```python
from build123d import *

# Parameters (mm, degrees)
F2_W     = 50.8
F2_H     = 76.2
F2_W_2   = 45.72
F2_H_2   = 71.12
F3_DEPTH = 50.8
F4_W     = 50.8
F4_H     = 76.2
F5_DEPTH = 2.54
F8_D     = 12.7
F8_DEPTH = 5.08
F8_TIP   = 3.8154649308


# Not quite as in the source:
# - a variable given as a bare number and used for a length is read in inches; the dataset says mm whatever the document's units were


with BuildPart() as f3:
    # F2 (on Top) → F3 (new body)
    with BuildSketch(Plane.XY):
        with Locations((25.4, 38.1)):
            Rectangle(F2_W, F2_H)
        with Locations((25.4, 38.1)):
            Rectangle(F2_W_2, F2_H_2, mode=Mode.SUBTRACT)
    extrude(amount=F3_DEPTH)

    # F4 (on Top) → F5 (join)
    with BuildSketch(Plane.XY):
        with Locations((25.4, 38.1)):
            Rectangle(F4_W, F4_H)
    extrude(amount=F5_DEPTH)

    # F8
    with Locations(Plane(origin=(0, 0, 0), x_dir=(0, -1, 0), z_dir=(-1, 0, 0))):
        with Locations((-14.4875170663, 10.56548208), (-32.958894968, 10.56548208), (-45.4774573445, 10.56548208), (-63.5905191302, 10.56548208)):
            Hole(F8_D / 2, depth=F8_DEPTH)
            with Locations((0, 0, -(F8_DEPTH + F8_TIP / 2))):  # 118° drill point
                Cone(0, F8_D / 2, F8_TIP, mode=Mode.SUBTRACT)


solid = f3.part
```
Here's how the part is built. I have some questions about the finished solid (model axes, mm). A direction names the side the tool comes from. Round coordinates to 2 decimals unless told otherwise and drop trailing zeros. Order: outer loops, then holes, each group sorted by start corner. A loop starts at its lowest first (then second) coordinate and runs counter-clockwise, first axis right, second up. Notation, with made-up numbers: M 30.25,-23 L 48.25,-23 A15 cw 48.25,2 Z; hole C 62.25,-9.5 d10. An arc over 180 degrees is marked long. One line per question, with ' | ' between items.
1) For faces 4 (the face through (0, 38, 25)), 5 (the face through (2.54, 38, 32)), 6 (the face through (1.29, 51.82, 10.3)), which set-ups out of +Z, -Z, +X, -X, +Y, -Y let a thin tool reach every point of the face, with its end or its side?
Working result:
face 4: +Z, -Z, -X, +Y, -Y | face 5: +Z | face 6: -X
2) I need wall thicknesses on line 1 along X through (y, z) = (70, 33); line 2 along Y through (x, z) = (23, 34.5); line 3 along Z through (x, y) = (10, 71). Which ranges of each line are inside material? Lowest first, please.
Working result:
line 1: 0 to 2.54, 48.26 to 50.8 | line 2: 0 to 2.54, 73.66 to 76.2 | line 3: 0 to 2.54
3) I want a section at C-C, the plane x = 42.5. Write out the boundary of the cut face in (y, z), then the cut area to 3 significant figures.
Working result:
outline: M 0,0 L 76.2,0 L 76.2,50.8 L 73.66,50.8 L 73.66,2.54 L 2.54,2.54 L 2.54,50.8 L 0,50.8 Z | area: 439 mm²
4) I want a section at D-D, the plane z = 13. Write out the boundary of the cut face in (x, y), then the cut area to 3 significant figures.
Working result:
outline: M 0,0 L 50.8,0 L 50.8,76.2 L 0,76.2 L 0,69.46 L 2.54,69.46 L 2.54,73.66 L 48.26,73.66 L 48.26,2.54 L 2.54,2.54 L 2.54,8.62 L 0,8.62 Z; M 0,20.35 L 2.54,20.35 L 2.54,27.09 L 0,27.09 Z; M 0,38.82 L 2.54,38.82 L 2.54,39.61 L 0,39.61 Z; M 0,51.34 L 2.54,51.34 L 2.54,57.73 L 0,57.73 Z | area: 500 mm²
5) I want a section at A-A, the plane z = 20.5. Write out the boundary of the cut face in (x, y).
Working result:
outline: M 0,0 L 50.8,0 L 50.8,76.2 L 0,76.2 Z; hole M 2.54,2.54 L 48.26,2.54 L 48.26,73.66 L 2.54,73.66 Z
6) I want a section at B-B, the plane y = 33. Write out the boundary of the cut face in (x, z).
Working result:
outline: M 0,0 L 50.8,0 L 50.8,50.8 L 48.26,50.8 L 48.26,2.54 L 2.54,2.54 L 2.54,4.22 L 0,4.22 Z; M 0,16.92 L 2.54,16.92 L 2.54,50.8 L 0,50.8 Z
7) If we mould it in two halves opening along Z, with no side actions, what happens to faces 1 (the face through (50.8, 38, 25)), 2 (the face through (1.29, 13.66, 16.86)), 3 (the face through (25, 39, 0))? For each: +Z half, -Z half, draft (parallel to the pull), parting line (faces both ways), or undercut.
Working result:
face 1: draft | face 2: undercut | face 3: -Z half
8) For pin 1 Ø2 at (x, y) = (15, 24) entering from +Z; pin 2 Ø7.5 at (y, z) = (32.96, 10.57) entering from -X, each with a flat end and sliding along its axis, tell me the tip position at first contact or that it passes through.
Working result:
pin 1: z = 2.54 | pin 2: x = 48.26
